Design review of the part built by this model. Coordinates are the model's own, in mm. Face numbers are marked on the shaded views. A direction names the side the tool comes from. Coordinates: 2 decimals unless noted, no trailing zeros. Order: outer loops, then holes, each group sorted by start corner. A loop starts at its lowest first (then second) coordinate and runs counter-clockwise, first axis right, second up. Notation, with made-up numbers: M -28.5,12.25 L -24.5,12.25 A17 cw -24.5,36.25 Z; hole C 3,28.5 d1. An arc over 180 degrees is marked long. Use CSV: the item, a comma, the result in double quotes.
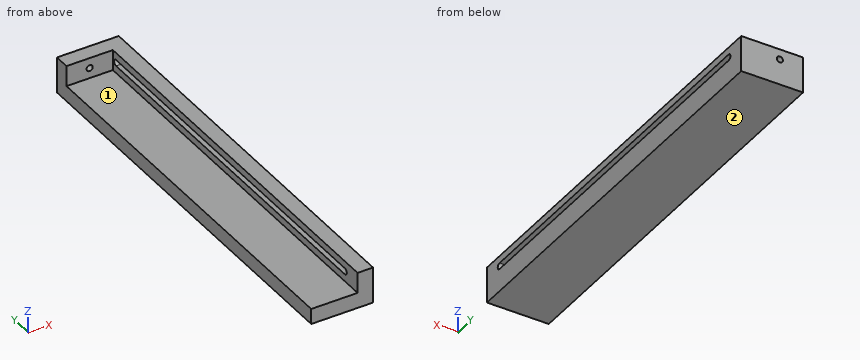
```python
from build123d import *

# Parameters (mm, degrees)
F0_W     = 60
F0_H     = 15
F1_DEPTH = 200
F2_W     = 15
F2_H     = 20
F3_DEPTH = 400
F5_DEPTH = 15.001
F6_W     = 45
F6_H     = 15
F7_DEPTH = 20
F8_R     = 3
F9_DEPTH = 15.001


with BuildPart() as f1:
    # F0 (on Front) → F1 (new body, symmetric)
    with BuildSketch(Plane.XZ):
        Rectangle(F0_W, F0_H)
    extrude(amount=F1_DEPTH, both=True)

    # F2 (on face) → F3 (join, through all)
    with BuildSketch(Plane.XZ.offset(200)):
        with Locations((22.5, 17.5)):
            Rectangle(F2_W, F2_H)
    extrude(amount=-F3_DEPTH)

    # F4 (on face) → F5 (cut, through all)
    with BuildSketch(Plane(origin=(15, 0, 0), x_dir=(0, -1, 0), z_dir=(-1, 0, 0))):
        with BuildLine():
            ThreePointArc((180, 14.5), (183, 17.5), (180, 20.5))
            Line((180, 20.5), (-180, 20.5))
            ThreePointArc((-180, 20.5), (-183, 17.5), (-180, 14.5))
            Line((-180, 14.5), (180, 14.5))
        make_face()
    extrude(amount=-F5_DEPTH, mode=Mode.SUBTRACT)

    # F6 (on face) → F7 (join)
    with BuildSketch(Plane.XY.offset(7.5)):
        with Locations((-7.5, 192.5)):
            Rectangle(F6_W, F6_H)
    extrude(amount=F7_DEPTH)

    # F8 (on face) → F9 (cut, through all)
    with BuildSketch(Plane.XZ.offset(-185)):
        with Locations((-7.5, 17.5)):
            Circle(F8_R)
    extrude(amount=-F9_DEPTH, mode=Mode.SUBTRACT)


solid = f1.part
```
(1) Add section B-B on x = 0.5. State the section outline as (y, z) points.
The answers:
outline,"M -200,-7.5 L 200,-7.5 L 200,27.5 L 185,27.5 L 185,7.5 L -200,7.5 Z"
(2) For the marked faces 1 and 2, list the 3-axis set-ups (+Z, -Z, +X, -X, +Y, -Y) from which the entire face can be reached by the end or side of a thin tool; tool diameter is ignored.
The answers:
face 1,"+Z, -X, -Y"
face 2,"-Z, +X, -X, +Y, -Y"
(3) Add section A-A on y = -65. State the section outline as (x, z) points, and give its area (3 significant figures).
The answers:
outline,"M -30,-7.5 L 30,-7.5 L 30,14.5 L 15,14.5 L 15,7.5 L -30,7.5 Z; M 15,20.5 L 30,20.5 L 30,27.5 L 15,27.5 Z"
area,"1,110 mm2"
(4) Wall thickness on probe 1 along Z at (x, y) = (23, 120.5); probe 2 along Z at (x, y) = (-26.5, -109); probe 3 along X at (y, z) = (-103.5, 22.5): over which ranges is each line inside the solid? List them lowest first.
The answers:
probe 1,"z = -7.5 to 14.5, 20.5 to 27.5"
probe 2,"z = -7.5 to 7.5"
probe 3,"x = 15 to 30"
(5) Clearance check with flat-ended pins moving along their axes: P1, Ø16, axis at x = 1, z = 13, coming from the -Y side; P2, Ø8, axis at x = -7.5, z = 17.5, coming from the -Y side; P3, Ø1.5, axis at y = -46.5, z = 18.5, coming from the +X side; P4, Ø10, axis at y = 51.5, z = 17, coming from the -X side. State where each tip first meets the part, or that it passes through.
The answers:
P1,"stops at y = -200"
P2,"stops at y = 185"
P3,"passes through"
P4,"stops at x = 15"
